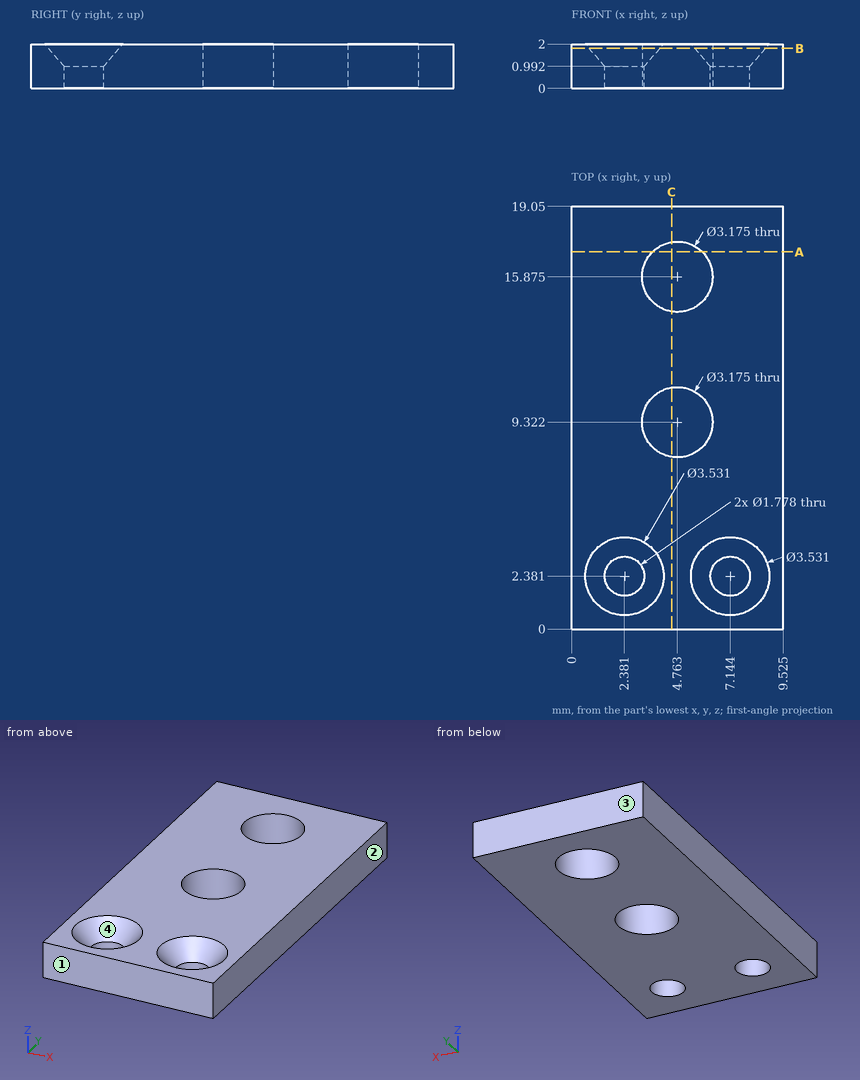
Geometry check sheet. Reference: drawing and pictorial views, mm from the part's lowest x, y, z. Give positions to 0.01 mm unless a question says otherwise; leave off trailing zeros. Loops run counter-clockwise (first coordinate to the right, second up) from the corner with the lowest first, then second, coordinate; pieces in that order, holes last.
1. Thickness scan on line 1 (X direction, y = 16, z = 0.65) (1 decimal); line 2 (X direction, y = 2, z = 0.55) (1 decimal); line 3 (X direction, y = 10.75, z = 0.7) (1 decimal). Record the ranges inside material, lowest first.
2. Section check C-C, the plane x = 4.5. Enter the section's corners in (y, z).
3. Section check A-A, the plane y = 17. Enter the section's corners in (x, z) (1 decimal).
4. Section check B-B, the plane z = 1.8. Count the separate pieces of the cut face and the enclosed holes in it, then the cut area to 3 significant figures.
5. Go/stop test with a flat-tipped pin: pin 1 Ø3 at (x, y) = (7.14, 2.38) entering from +Z. Record where the tip stops, or that it passes through.
6. Mould release check, pull along Y, two halves, no side actions. Record for the marked faces 1, 2, 3 and 4: released by +Y, released by -Y, zero draft, split by the parting line, or undercut.
Geometry says:
1. line 1: x = 0 to 3.2, 6.3 to 9.5
1. line 2: x = 0 to 1.6, 3.2 to 6.3, 7.9 to 9.5
1. line 3: x = 0 to 4.1, 5.5 to 9.5
2. outline: (0, 0) - (7.76, 0) - (7.76, 2) - (0, 2) - close; (10.89, 0) - (14.31, 0) - (14.31, 2) - (10.89, 2) - close; (17.44, 0) - (19.05, 0) - (19.05, 2) - (17.44, 2) - close
3. outline: (0, 0) - (3.6, 0) - (3.6, 2) - (0, 2) - close; (5.9, 0) - (9.5, 0) - (9.5, 2) - (5.9, 2) - close
4. separate pieces: 1
4. enclosed holes: 4
4. area: 150 mm2
5. pin 1: stops at z = 1.7
6. face 1: released by -Y
6. face 2: zero draft
6. face 3: released by +Y
6. face 4: undercut
